from build123d import *

# Parameters (mm, degrees)
SKETCH_1_R          = 1.6
SKETCH_1_R_2        = 12.5
EXTRUDE_1_DEPTH     = 5
SKETCH_2_W          = 50
SKETCH_2_H          = 3.896696611
EXTRUDE_2_DEPTH     = 25
SKETCH_3_R          = 1.6
CUT_EXTRUDE_1_DEPTH = 25


with BuildPart() as part:
    # 草图1 → 凸台-拉伸1 (new body)
    with BuildSketch(Plane.XY):
        with BuildLine():
            Line((-25, -22), (25, -22))
            Line((25, -22), (25, -18.103303389))
            Line((25, -18.103303389), (17.666287953, 5.491108263))
            ThreePointArc((17.666287953, 5.491108263), (0, 18.5), (-17.666287953, 5.491108263))
            Line((-17.666287953, 5.491108263), (-25, -18.103303389))
            Line((-25, -18.103303389), (-25, -22))
        make_face()
        with Locations((-15.5, 0)):
            Circle(SKETCH_1_R, mode=Mode.SUBTRACT)
        with Locations((-7.75, 13.423393759)):
            Circle(SKETCH_1_R, mode=Mode.SUBTRACT)
        with Locations((7.75, 13.423393759)):
            Circle(SKETCH_1_R, mode=Mode.SUBTRACT)
        with Locations((15.5, 0)):
            Circle(SKETCH_1_R, mode=Mode.SUBTRACT)
        with Locations((7.75, -13.423393759)):
            Circle(SKETCH_1_R, mode=Mode.SUBTRACT)
        with Locations((-7.75, -13.423393759)):
            Circle(SKETCH_1_R, mode=Mode.SUBTRACT)
        Circle(SKETCH_1_R_2, mode=Mode.SUBTRACT)
    extrude(amount=EXTRUDE_1_DEPTH)

    # 草图2 → 凸台-拉伸2 (add)
    with BuildSketch(Plane(origin=(0, 0, 0), x_dir=(-1, 0, 0), z_dir=(0, 0, -1))):
        with Locations((0, -20.051651695)):
            Rectangle(SKETCH_2_W, SKETCH_2_H)
    extrude(amount=EXTRUDE_2_DEPTH)

    # 草图3 → 切除-拉伸1 (cut)
    with BuildSketch(Plane(origin=(0, -18.103303389, 0), x_dir=(1, 0, 0), z_dir=(0, 1, 0))):
        with Locations((-20, 20)):
            Circle(SKETCH_3_R)
        with Locations((20, 20)):
            Circle(SKETCH_3_R)
        with Locations((20, 5)):
            Circle(SKETCH_3_R)
        with Locations((-20, 5)):
            Circle(SKETCH_3_R)
    extrude(amount=-CUT_EXTRUDE_1_DEPTH, mode=Mode.SUBTRACT)


solid = part.part
Source: CAD feature listing. Evaluate the final solid. Frame: model axes, mm. A direction names the side the tool comes from. Round coordinates to 2 decimals unless told otherwise and drop trailing zeros. Loops run counter-clockwise (first coordinate to the right, second up) from the corner with the lowest first, then second, coordinate; pieces in that order, holes last.
Q1. Section C-C, the plane x = 20. Return loops of the section in (y, z).
Q2. Ray query, line 1 (Z direction, x = 20, y = -21); line 2 (X direction, y = -19.75, z = -20); line 3 (Y direction, x = 7.75, z = 3.9). Return the intervals inside material, ascending.
Q3. Section B-B, the plane x = 2.5. Return loops of the section in (y, z), plus the area to 3 significant figures.
Q4. First-contact query: P1, Ø1.9, axis at x = -7.75, y = -13.42, coming from the -Z side; P2, Ø3.5, axis at x = 15.5, y = 0, coming from the -Z side; P3, Ø5, axis at x = -20, z = -5, coming from the +Y side; P4, Ø3.5, axis at x = 7.75, y = 13.42, coming from the +Z side. Flat tips, straight axial feed; report the tip coordinate or a pass-through.
Q5. Mould query, pull axis Y, two halves, no side actions, for faces 3 (the face through (25, -20, -10)), 4 (the face through (7.403, -14.985, 2.465)), 5 (the face through (0, -22, -10)), 6 (the face through (-8.097, -14.985, 2.465)). Classes: pulls with the +Y half, pulls with the -Y half, needs draft (parallel to the pull), parting line crosses it, or undercut.
Q6. Section A-A, the plane z = -5. Return loops of the section in (x, y), plus the area to 3 significant figures.
Q7. Section D-D, the plane y = 2.5. Return loops of the section in (x, z), plus the area to 3 significant figures.
Q8. Access query for faces 1 (the face through (0, -20, -25)), 2 (the face through (0, -18.103, -12)). Directions: +Z, -Z, +X, -X, +Y, -Y. A direction counts if a zero-diameter tool reaches every point of the face in a straight line with its end or side. Return the directions, or none.
Solutions:
1. outline: (-22, -25) - (-18.1, -25) - (-18.1, -21.6) - (-22, -21.6) - close; (-22, -18.4) - (-18.1, -18.4) - (-18.1, -6.6) - (-22, -6.6) - close; (-22, -3.4) - (-18.1, -3.4) - (-18.1, 0) - (-2.02, 0) - (-2.02, 5) - (-22, 5) - close
2. line 1: z = -25 to -21.6, -18.4 to -6.6, -3.4 to 5
2. line 2: x = -25 to -21.6, -18.4 to 18.4, 21.6 to 25
2. line 3: y = -22 to -15.02, -11.82 to -9.81, 9.81 to 11.82, 15.02 to 16.8
3. outline: (-22, -25) - (-18.1, -25) - (-18.1, 0) - (-12.25, 0) - (-12.25, 5) - (-22, 5) - close; (12.25, 0) - (18.33, 0) - (18.33, 5) - (12.25, 5) - close
3. area: 177 mm2
4. P1: passes through
4. P2: stops at z = 0
4. P3: stops at y = -18.1
4. P4: stops at z = 5
5. face 3: needs draft
5. face 4: undercut
5. face 5: pulls with the -Y half
5. face 6: undercut
6. outline: (-25, -22) - (-21.6, -22) - (-21.6, -18.1) - (-25, -18.1) - close; (-18.4, -22) - (18.4, -22) - (18.4, -18.1) - (-18.4, -18.1) - close; (21.6, -22) - (25, -22) - (25, -18.1) - (21.6, -18.1) - close
6. area: 170 mm2
7. outline: (-18.6, 0) - (-12.25, 0) - (-12.25, 5) - (-18.6, 5) - close; (12.25, 0) - (18.6, 0) - (18.6, 5) - (12.25, 5) - close
7. area: 63.5 mm2
8. face 1: -Z, +X, -X, +Y, -Y
8. face 2: -Z, +X, -X, +Y
